Input: dimensioned drawing with shaded views. Units: mm. Origin: part minimum x, y, z. Round coordinates to 2 decimals unless told otherwise and drop trailing zeros. Order: outer loops, then holes, each group sorted by start corner. A loop starts at its lowest first (then second) coordinate and runs counter-clockwise, first axis right, second up. Notation, with made-up numbers: M 70.5,15 L 104.5,15 A16 ccw 104.5,28 Z; hole C 73,-31.5 d9. An arc over 180 degrees is marked long. Use CSV: the item, a comma, the result in double quotes. Start each with the question number.
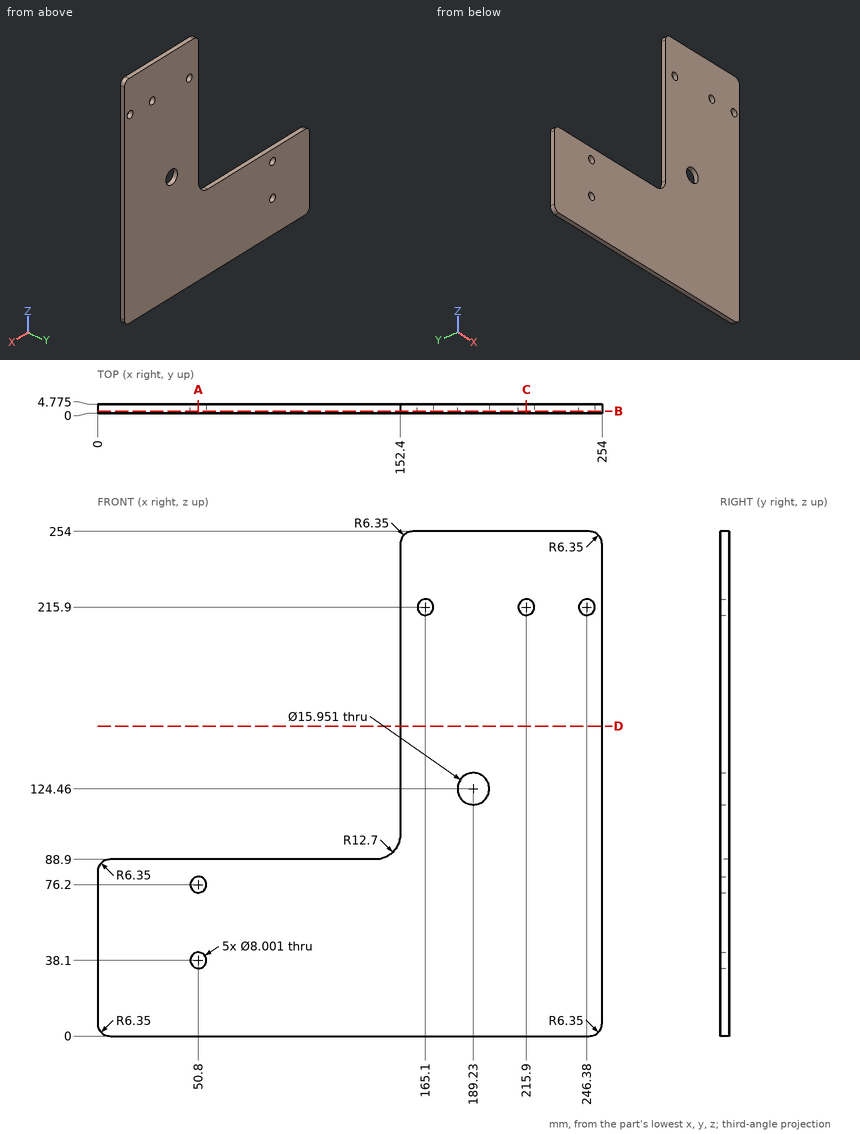
(1) Section B-B on y = 1.2. Return loops of the section in (x, z).
(2) Section C-C on x = 215.9. Return loops of the section in (y, z) (1 decimal), plus the area to 3 significant figures.
(3) Line query: line 1 along Z through (x, y) = (50.8, 3.65); line 2 along Z through (x, y) = (189.23, 1.2); line 3 along Z through (x, y) = (54, 0.6). Output: solid intervals per line, ascending.
(4) Contact query for flat-ended pins moving along their axis: P1, Ø14.5, axis at x = 189.23, z = 124.46, coming from the +Y side; P2, Ø1.4, axis at x = 61.5, y = 1.5, coming from the +Z side; P3, Ø1.4, axis at y = 2, z = 203.5, coming from the -X side. Output: stop coordinate, or through.
(5) Section D-D on z = 156. Return loops of the section in (x, y) (1 decimal), plus the area to 3 significant figures.
(6) Section A-A on x = 50.8. Return loops of the section in (y, z) (1 decimal).
Results below:
1,outline,"M 0,6.35 A6.35 ccw 6.35,0 L 247.65,0 A6.35 ccw 254,6.35 L 254,247.65 A6.35 ccw 247.65,254 L 158.75,254 A6.35 ccw 152.4,247.65 L 152.4,101.6 A12.7 cw 139.7,88.9 L 6.35,88.9 A6.35 ccw 0,82.55 Z; hole C 50.8,38.1 d8; hole C 50.8,76.2 d8; hole C 165.1,215.9 d8; hole C 189.23,124.46 d15.95; hole C 215.9,215.9 d8; hole C 246.38,215.9 d8"
2,outline,"M 0,0 L 4.8,0 L 4.8,211.9 L 0,211.9 Z; M 0,219.9 L 4.8,219.9 L 4.8,254 L 0,254 Z"
2,area,"1,170 mm2"
3,line 1,"z = 0 to 34.1, 42.1 to 72.2, 80.2 to 88.9"
3,line 2,"z = 0 to 116.48, 132.44 to 254"
3,line 3,"z = 0 to 35.7, 40.5 to 73.8, 78.6 to 88.9"
4,P1,"passes through"
4,P2,"stops at z = 88.9"
4,P3,"stops at x = 152.4"
5,outline,"M 152.4,0 L 254,0 L 254,4.8 L 152.4,4.8 Z"
5,area,"485 mm2"
6,outline,"M 0,0 L 4.8,0 L 4.8,34.1 L 0,34.1 Z; M 0,42.1 L 4.8,42.1 L 4.8,72.2 L 0,72.2 Z; M 0,80.2 L 4.8,80.2 L 4.8,88.9 L 0,88.9 Z"
